Input: part model. Units: mm. Frame: model coordinates. Face numbers are marked on the shaded views. A direction names the side the tool comes from. Round coordinates to 2 decimals unless told otherwise and drop trailing zeros. Write each loop counter-clockwise with the first axis right and the second up, starting at its lowest first coordinate (ties: lowest second). Pieces come first, ordered by that corner, then holes. Notation, with made-up numbers: M 54,69.25 L 70,69.25 A26 cw 70,96.25 Z; hole C 88.5,73.25 d6. An arc over 180 degrees is marked long. Use one line per item in the form item = value. Start each with the question number.
Autodesk Inventor part; units mm, degrees
ref_plane "YZ Plane" through (0, 0, 0) normal (1, 0, 0) x (0, 1, 0)
ref_plane "XZ Plane" through (0, 0, 0) normal (0, 1, 0) x (-1, 0, 0)
ref_plane "XY Plane" through (0, 0, 0) normal (0, 0, 1) x (1, 0, 0)
sketch "Sketch1" plane through (0, 0, 0) normal (0, 0, 1) x (1, 0, 0)
  line L0 (-9.9228, 0) -> (-13.5328, 0)
  line L1 (-13.5328, 0) -> (-13.5328, 4)
  line L2 (-13.5328, 4) -> (-9.9228, 4)
  line L3 (-9.9228, 4) -> (-9.9228, 0)
  line L4 (-9.9228, 0) -> (-9.9228, -45)
  line L5 (-9.9228, -45) -> (-11.9228, -45)
  line L6 (-11.9228, -45) -> (-11.9228, 0)
  point P0 (0, 0)
  dimension "d0" = 3.61
  dimension "d1" = 4
  dimension "d2" = 45
  dimension "d3" = 2
revolve "Revolution1" add sketch "Sketch1" angle 360 about axis through (-9.9228, 0, 0) along (0, -1, 0)
chamfer "Chamfer1" distance 0.4 angle 45 1 edges at (-6.3128, 4, 0)
sketch "Boceto2" plane through (-9.9228, 4, 0) normal (0, 1, 0) x (1, 0, 0)
  line L0 (1.1641, -1.3443) -> (-0.5821, -1.6803)
  line L1 (-0.5821, -1.6803) -> (-1.7462, -0.336)
  line L2 (-1.7462, -0.336) -> (-1.1641, 1.3443)
  line L3 (-1.1641, 1.3443) -> (0.5821, 1.6803)
  line L4 (0.5821, 1.6803) -> (1.7462, 0.336)
  line L5 (1.7462, 0.336) -> (1.1641, -1.3443)
  point P0 (9.9228, 0)
  point P1 (0, 0)
  dimension "d11" = 3.08
extrude "Extrusión1" cut sketch "Boceto2" against normal blind 2
thread "Rosca1"
properties part number "Tornillo Allen cabeza cilindrica M4x50mm"
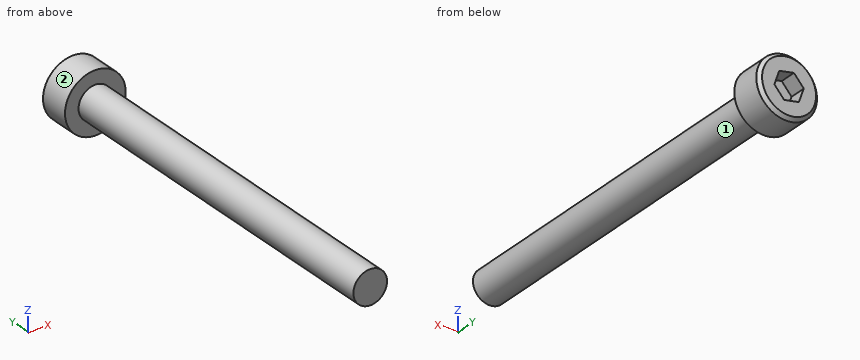
Item 1: First-contact query: pin 1 (3 mm diameter, centred on y = -37, z = 0.5, fed in from -X); pin 2 (1 mm diameter, centred on x = -10, y = -8, fed in from -Z); pin 3 (1 mm diameter, centred on x = -8, y = -13, fed in from +Z). Flat tips, straight axial feed; report the tip coordinate or a pass-through.
Item 2: Reachability of the marked faces 1 and 2 from +Z, -Z, +X, -X, +Y, -Y: full face, straight path, thin tool, end or side. Return the list, or none.
Item 3: Cut plane A-A (y = -23). Output: boundary loops of the cut face in (x, z).
Item 4: Ray query, line 1 (Y direction, x = -11.25, z = 0); line 2 (Z direction, x = -10, y = -43); line 3 (Y direction, x = -8.5, z = 1.75). Return the intervals inside material, ascending. Write a range as from..to.
Final values:
q1.pin_1 = -11.92
q1.pin_2 = -2
q1.pin_3 = 1.41
q2.face_1 = -Y
q2.face_2 = +Y, -Y
q3.outline = C -9.92,0 d4
q4.line_1 = -45..2
q4.line_2 = -2..2
q4.line_3 = 0..4
